Read the model definition and answer for the solid it produces. Units are mm, in the model's axes. Face numbers are marked on the shaded views. Give positions to 0.01 mm unless a question says otherwise; leave off trailing zeros. Loops run counter-clockwise (first coordinate to the right, second up) from the corner with the lowest first, then second, coordinate; pieces in that order, holes last. Notation, with made-up numbers: (-23.75, -2.75) -> (11.25, -2.75) arc R24 cw to (11.25, 15.25) -> close; hole circle Ø10 at (65, 18.5). An arc over 180 degrees is marked (long way). Return JSON: item names as keys, results as strings. Group by question number.
from build123d import *

# Parameters (mm, degrees)
F1_DEPTH     = 6
F3_DEPTH     = 3
F4_R         = 12.5
F5_DEPTH     = 25
F6_R         = 1.75
F7_DEPTH     = 25
F8_R         = 1.75
F9_DEPTH     = 25
F10_T1_DEPTH = 6
F10_T3_DEPTH = 3
F11_R        = 2


# Not quite as in the source:
# - a fillet or chamfer that OpenCascade refuses, or shapes differently, is made with other operations: its cross-section is extruded or revolved along the edge and cut away or added


with BuildPart() as f1:
    # F0 (on Top) → F1 (new body)
    with BuildSketch(Plane.XY):
        Polygon((15.5, -15.5), (0, -15.5), (0, -100.5), (15.5, -100.5), (15.5, -116), (54.5, -116), (54.5, -100.5), (70, -100.5), (70, -15.5), (54.5, -15.5), (54.5, 0), (15.5, 0), align=None)
    extrude(amount=F1_DEPTH)

    # F2 (on face) → F3 (cut)
    with BuildSketch(Plane(origin=(0, 0, 0), x_dir=(1, 0, 0), z_dir=(0, 0, -1))):
        with BuildLine():
            Line((46.0390912639, 107.6606247352), (48.3088987836, 107.6606247352))
            ThreePointArc((48.3088987836, 107.6606247352), (47.1739950237, 107.6916095092), (46.0390912639, 107.6606247352))
        make_face()
        with BuildLine():
            Line((46.863162711, 63.6384694919), (48.4956821186, 63.6384694919))
            ThreePointArc((48.4956821186, 63.6384694919), (47.6794224148, 63.6544920069), (46.863162711, 63.6384694919))
        make_face()
        with BuildLine():
            Line((54.5, 107.6606247352), (48.3088987836, 107.6606247352))
            Line((48.3088987836, 107.6606247352), (46.0390912639, 107.6606247352))
            ThreePointArc((46.0390912639, 107.6606247352), (26.3780814544, 86.4793246358), (46.863162711, 66.0939321564))
            Line((46.863162711, 66.0939321564), (70, 66.0939321564))
            Line((70, 66.0939321564), (70, 100.5))
            Line((70, 100.5), (54.5, 100.5))
            Line((54.5, 100.5), (54.5, 107.6606247352))
        make_face()
        with BuildLine():
            Line((70, 22.1093658845), (70, 63.6384694919))
            Line((70, 63.6384694919), (48.4956821186, 63.6384694919))
            Line((48.4956821186, 63.6384694919), (46.863162711, 63.6384694919))
            ThreePointArc((46.863162711, 63.6384694919), (26.8823229814, 43.2018465212), (46.1695409076, 22.1093658845))
            Line((46.1695409076, 22.1093658845), (70, 22.1093658845))
        make_face()
    extrude(amount=-F3_DEPTH, mode=Mode.SUBTRACT)

    # F4 (on face) → F5 (cut)
    with BuildSketch(Plane(origin=(0, 0, 3), x_dir=(1, 0, 0), z_dir=(0, 0, -1))):
        with Locations((47.51990363, 42.9035276175)):
            Circle(F4_R)
        with Locations((47.1739950237, 86.8916095092)):
            Circle(F4_R)
    extrude(amount=-F5_DEPTH, mode=Mode.SUBTRACT)

    # F6 (on face) → F7 (cut)
    with BuildSketch(Plane(origin=(0, 0, 3), x_dir=(1, 0, 0), z_dir=(0, 0, -1))):
        with Locations((39.0656358559, 58.0877674629)):
            Circle(F6_R)
        with Locations((30.1801256076, 43.0113717521)):
            Circle(F6_R)
        with Locations((38.7939121665, 27.7780962961)):
            Circle(F6_R)
        with Locations((56.2932089737, 27.6212165509)):
            Circle(F6_R)
        with Locations((65.178719222, 42.6976122617)):
            Circle(F6_R)
        with Locations((56.5649326631, 57.9308877176)):
            Circle(F6_R)
    extrude(amount=-F7_DEPTH, mode=Mode.SUBTRACT)

    # F8 (on face) → F9 (cut)
    with BuildSketch(Plane(origin=(0, 0, 3), x_dir=(1, 0, 0), z_dir=(0, 0, -1))):
        with Locations((35.8538748382, 100.2372035006)):
            Circle(F8_R)
        with Locations((29.9563115058, 83.7608948503)):
            Circle(F8_R)
        with Locations((41.2764316914, 70.4153008589)):
            Circle(F8_R)
        with Locations((58.4941152093, 73.5460155178)):
            Circle(F8_R)
        with Locations((64.3916785417, 90.0223241681)):
            Circle(F8_R)
        with Locations((53.0715583561, 103.3679181595)):
            Circle(F8_R)
    extrude(amount=-F9_DEPTH, mode=Mode.SUBTRACT)

    # F10: fillet of radius 2 on 2 edges, made by hand

    # F10_s2 → F10_t1 (join)
    with BuildSketch(Plane.XY):
        with BuildLine():
            ThreePointArc((13.5, -100.5), (14.9142135624, -101.0857864376), (15.5, -102.5))
            Line((15.5, -102.5), (15.5, -100.5))
            Line((15.5, -100.5), (13.5, -100.5))
        make_face()
    extrude(amount=F10_T1_DEPTH)

    # F10_s4 → F10_t3 (join)
    with BuildSketch(Plane.XY.offset(3)):
        with BuildLine():
            ThreePointArc((56.4948776909, -100.5), (55.1321777741, -101.0360843819), (54.5, -102.3569510631))
            Line((54.5, -102.3569510631), (54.5, -100.5))
            Line((54.5, -100.5), (56.4948776909, -100.5))
        make_face()
    extrude(amount=F10_T3_DEPTH)

    # F11
    f11_edges = [f1.edges().sort_by_distance(p)[0] for p in [
        (54.5, -15.5, 3),
        (15.5, -15.5, 3),
    ]]
    fillet(f11_edges, radius=F11_R)


solid = f1.part
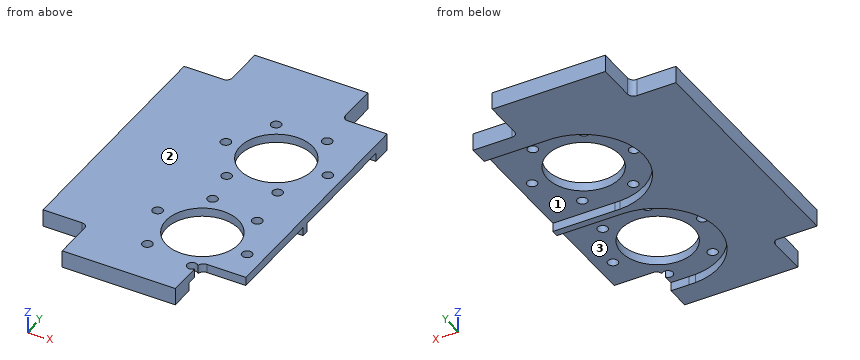
1. Flat-ended cylindrical pins translate along their axes: pin 1 Ø5.5 at (x, y) = (41.28, -70.42) entering from -Z; pin 2 Ø0.9 at (x, z) = (58.5, 1) entering from +Y. Find the tip coordinate at first contact, or state that the pin passes through.
2. Determine the mould class of the marked faces 1, 2 and 3 for opening direction Y: pulls with the +Y half, pulls with the -Y half, needs draft (parallel to the pull), parting line crosses it, or undercut.
3. Section B-B on x = 30.5 is taken. Determine the outline of the cut face in (y, z), then the cut area to 3 significant figures.
4. Section D-D on y = -7 is taken. Determine the outline of the cut face in (x, z), then the cut area to 3 significant figures.
5. Section C-C on z = 4.2 is taken. State how many separate pieces and enclosed holes the cut face has, then the cut area to 3 significant figures.
6. Section A-A on y = -49 is taken. Determine the outline of the cut face in (x, z).
7. Straight lines are drawn through the part: line 1 (Y direction, x = 49, z = 2.3); line 2 (Y direction, x = 54, z = 5.35); line 3 (Y direction, x = 56.5, z = 2.1). For each, find the intervals that lie inside material, in ascending order. Write a range as from..to.
Completed:
{
 "1": {"pin 1": "stops at z = 3", "pin 2": "stops at y = -15.5"},
 "2": {"face 1": "undercut", "face 2": "needs draft", "face 3": "undercut"},
 "3": {"outline": "(-116, 0) -> (-99.33, 0) -> (-99.33, 3) -> (-85.42, 3) -> (-85.42, 6) -> (-116, 6) -> close; (-82.1, 3) -> (-74.46, 3) -> (-74.46, 0) -> (-54.58, 0) -> (-54.58, 3) -> (-44.73, 3) -> (-44.73, 6) -> (-82.1, 6) -> close; (-41.29, 3) -> (-31.13, 3) -> (-31.13, 0) -> (0, 0) -> (0, 6) -> (-41.29, 6) -> close", "area": "531 mm²"},
 "4": {"outline": "(15.5, 0) -> (54.5, 0) -> (54.5, 6) -> (15.5, 6) -> close", "area": "234 mm²"},
 "5": {"separate pieces": "1", "enclosed holes": "13", "area": "6,070 mm²"},
 "6": {"outline": "(0, 0) -> (27.81, 0) -> (27.81, 3) -> (36.61, 3) -> (36.61, 6) -> (0, 6) -> close; (58.43, 3) -> (70, 3) -> (70, 6) -> (58.43, 6) -> close"},
 "7": {"line 1": "y = -116..-107.66, -66.09..-63.64, -22.11..0", "line 2": "y = -116..-104.85, -101.88..-97.36, -76.42..-53.59, -32.21..0", "line 3": "y = -66.09..-63.64, -22.11..-15.5"}
}
